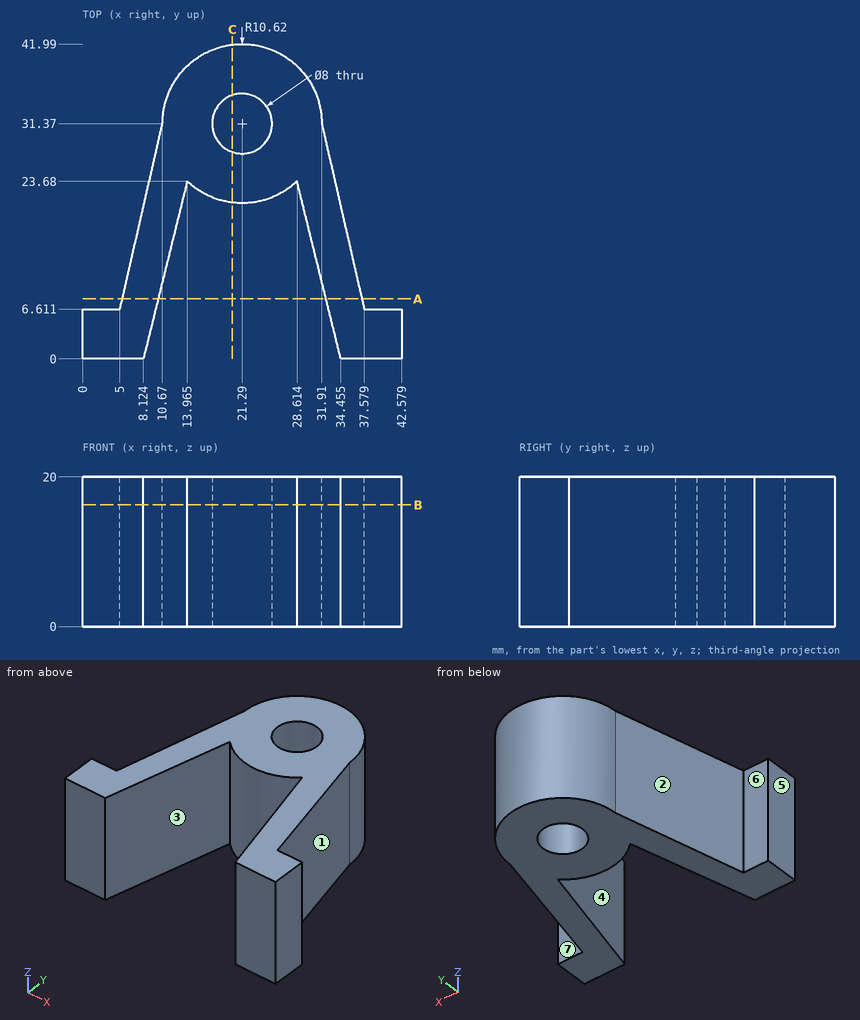
Could you check a few things on this drawing? It's one solid part, dimensions in mm from its lowest x, y, z. A direction names the side the tool comes from. Round coordinates to 2 decimals unless told otherwise and drop trailing zeros. Write each loop counter-clockwise with the first axis right and the second up, starting at its lowest first coordinate (ties: lowest second). Pieces come first, ordered by that corner, then holes. Notation, with made-up numbers: M 8.25,4.25 L 50.25,4.25 A18 cw 50.25,10.25 Z; hole C 23.25,12 d10. An arc over 180 degrees is marked long. Answer as CSV lines item,"result". Start each with the question number.
1. Thinking about a two-plate mould opening in X: for the marked faces 1, 2, 3 and 4, which applies, released by +X, released by -X, zero draft, split by the parting line, or undercut?
2. Suppose I cut it at C-C on x = 20. Write out the boundary of the cut face in (y, z).
3. I'm going to push flat-ended pins straight in: pin 1 Ø12 at (x, z) = (20, 9) entering from -Y; pin 2 Ø3 at (x, z) = (24.5, 6) entering from -Y; pin 3 Ø10 at (y, z) = (37, 10) entering from -X. Where does each tip first touch, or does it pass through?
4. On a 3-axis mill with a long thin cutter (end or side, diameter ignored), from which of +Z, -Z, +X, -X, +Y, -Y can I reach the whole of each face in a straight line? I mean the marked faces 5, 6 and 7. Say none if no direction works.
5. Suppose I cut it at B-B on z = 16.25. Write out the boundary of the cut face in (x, y) (1 decimal), then the cut area to 3 significant figures.
6. I need wall thicknesses on probe 1 along X at (y, z) = (31.5, 6.75); probe 2 along Y at (x, z) = (23.5, 18) (1 decimal); probe 3 along Y at (x, z) = (20, 18) (1 decimal). Which ranges of each line are inside material? Lowest first, please.
7. Suppose I cut it at A-A on y = 8. Write out the boundary of the cut face in (x, z), then the cut area to 3 significant figures.
Check result:
1,face 1,"released by +X"
1,face 2,"released by -X"
1,face 3,"undercut"
1,face 4,"undercut"
2,outline,"M 20.83,0 L 27.58,0 L 27.58,20 L 20.83,20 Z; M 35.16,0 L 41.91,0 L 41.91,20 L 35.16,20 Z"
3,pin 1,"stops at y = 20.75"
3,pin 2,"stops at y = 20.89"
3,pin 3,"stops at x = 10.69"
4,face 5,"+Z, -Z, -X, +Y, -Y"
4,face 6,"+Z, -Z, -X, +Y"
4,face 7,"+Z, -Z, +X, +Y"
5,outline,"M 0,0 L 8.1,0 L 14,23.7 A10.6 ccw 28.6,23.7 L 34.5,0 L 42.6,0 L 42.6,6.6 L 37.6,6.6 L 31.9,31.4 A10.6 ccw 10.7,31.4 L 5,6.6 L 0,6.6 Z; hole C 21.3,31.4 d8"
5,area,"619 mm2"
6,probe 1,"x = 10.67 to 17.29, 25.29 to 31.91"
6,probe 2,"y = 21 to 28, 34.7 to 41.8"
6,probe 3,"y = 20.8 to 27.6, 35.2 to 41.9"
7,outline,"M 5.32,0 L 10.1,0 L 10.1,20 L 5.32,20 Z; M 32.48,0 L 37.26,0 L 37.26,20 L 32.48,20 Z"
7,area,"191 mm2"
